Work out the finished part from the listing and answer in its coordinate system (mm). Face numbers are marked on the shaded views. A direction names the side the tool comes from. Give positions to 0.01 mm unless a question says otherwise; leave off trailing zeros. Write each loop counter-clockwise with the first axis right and the second up, starting at its lowest first coordinate (ties: lowest second). Pieces come first, ordered by that corner, then holes. Notation, with made-up numbers: (-5, 19) - (44, 19) arc R21 cw to (44, 49) - close; hole circle Ø8 at (-32, 78). An arc over 180 degrees is marked (long way). Write each question's results on one line, items separated by ' | '. Start each with the question number.
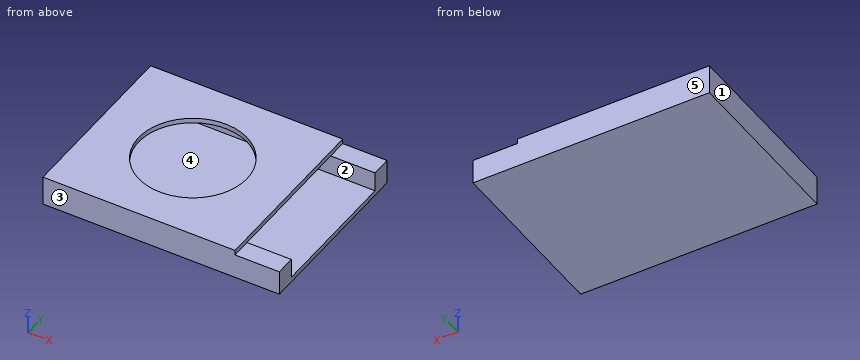
from build123d import *

# Parameters (mm, degrees)
F0_W     = 152.4
F0_H     = 114.3
F1_DEPTH = 3.175
F2_W     = 152.4
F2_H     = 12.7
F3_DEPTH = 12.7
F4_W     = 12.7
F4_H     = 88.9
F5_DEPTH = 12.7
F6_W     = 123.825
F6_H     = 114.3
F7_DEPTH = 3.175
F8_R     = 34.925
F9_DEPTH = 3.175


with BuildPart() as f1:
    # F0 (on Top) → F1 (new body)
    with BuildSketch(Plane.XY):
        Rectangle(F0_W, F0_H)
    extrude(amount=F1_DEPTH)

    # F2 (on face) → F3 (join)
    with BuildSketch(Plane.XY.offset(3.175)):
        with Locations((0, -50.8)):
            Rectangle(F2_W, F2_H)
        with Locations((0, 50.8)):
            Rectangle(F2_W, F2_H)
    extrude(amount=F3_DEPTH)

    # F4 (on face) → F5 (join)
    with BuildSketch(Plane.XY.offset(3.175)):
        with Locations((-69.85, 0)):
            Rectangle(F4_W, F4_H)
    extrude(amount=F5_DEPTH)

    # F6 (on face) → F7 (join)
    with BuildSketch(Plane.XY.offset(15.875)):
        with Locations((-14.2875, 0)):
            Rectangle(F6_W, F6_H)
    extrude(amount=F7_DEPTH)

    # F8 (on face) → F9 (cut)
    with BuildSketch(Plane.XY.offset(19.05)):
        with Locations((-14.2875, 0)):
            Circle(F8_R)
    extrude(amount=-F9_DEPTH, mode=Mode.SUBTRACT)


solid = f1.part
Q1. Given pin 1 (2 mm diameter, centred on x = -38, y = -1.5, fed in from -Z); pin 2 (2.5 mm diameter, centred on y = 6.5, z = 17, fed in from +X) (3 decimals); pin 3 (14 mm diameter, centred on x = 69, y = -54, fed in from +Z) (3 decimals); pin 4 (1 mm diameter, centred on y = 20.5, z = 5.5, fed in from +X), each flat-ended and moving along its own axis, determine where each tip first touches the part or whether it passes through.
Q2. A tool of negligible diameter and unlimited length cuts with its end or side. For the marked faces 4 and 5, from which of +Z, -Z, +X, -X, +Y, -Y can it reach the whole face along a straight path? Write none if from no direction.
Q3. A cutting plane is placed at B-B, the plane y = 8.5. Write down the section's boundary in (x, z) (3 decimals), and give its area (3 significant figures).
Q4. The mould has two halves that part along Y. Classify the marked faces 1, 2 and 3: pulls with the +Y half, pulls with the -Y half, needs draft (parallel to the pull), parting line crosses it, or undercut.
Q5. A cutting plane is placed at D-D, the plane y = 38. Write down the section's boundary in (x, z) (3 decimals), and give its area (3 significant figures).
Q6. A cutting plane is placed at C-C, the plane z = 10.75. Write down the section's boundary in (x, y), and give its area (3 significant figures).
Q7. A cutting plane is placed at A-A, the plane x = 44.5. Write down the section's boundary in (y, z) (3 decimals), and give its area (3 significant figures).
Q8. Consider L1, parallel to Y at x = 43, z = 11; L2, parallel to Z at x = -60, y = 41 (3 decimals); L3, parallel to Z at x = 54.5, y = -18.5 (3 decimals). Determine where each line is inside the solid, lowest interval first.
Result:
1) pin 1: stops at z = 0 | pin 2: stops at x = 47.625 | pin 3: stops at z = 15.875 | pin 4: stops at x = -63.5
2) face 4: +X | face 5: +Z, -Z, +X, -X, +Y
3) outline: (-76.2, 0) - (76.2, 0) - (76.2, 3.175) - (-63.5, 3.175) - (-63.5, 15.875) - (-48.162, 15.875) - (-48.162, 19.05) - (-76.2, 19.05) - close; (19.587, 15.875) - (47.625, 15.875) - (47.625, 19.05) - (19.587, 19.05) - close | area: 823 mm2
4) face 1: needs draft | face 2: undercut | face 3: pulls with the -Y half
5) outline: (-76.2, 0) - (76.2, 0) - (76.2, 3.175) - (-63.5, 3.175) - (-63.5, 15.875) - (47.625, 15.875) - (47.625, 19.05) - (-76.2, 19.05) - close | area: 1,040 mm2
6) outline: (-76.2, -57.15) - (76.2, -57.15) - (76.2, -44.45) - (-63.5, -44.45) - (-63.5, 44.45) - (76.2, 44.45) - (76.2, 57.15) - (-76.2, 57.15) - close | area: 5,000 mm2
7) outline: (-57.15, 0) - (57.15, 0) - (57.15, 19.05) - (-57.15, 19.05) - close; hole (-44.45, 3.175) - (44.45, 3.175) - (44.45, 15.875) - (-44.45, 15.875) - close | area: 1,050 mm2
8) L1: y = -57.15 to -44.45, 44.45 to 57.15 | L2: z = 0 to 3.175, 15.875 to 19.05 | L3: z = 0 to 3.175
